Can you work these out from the drawing? Everything is in mm from the part's minimum corner. A direction names the side the tool comes from. Coordinates: 2 decimals unless noted, no trailing zeros. Loops run counter-clockwise (first coordinate to the right, second up) from the corner with the lowest first, then second, coordinate; pieces in that order, holes last.
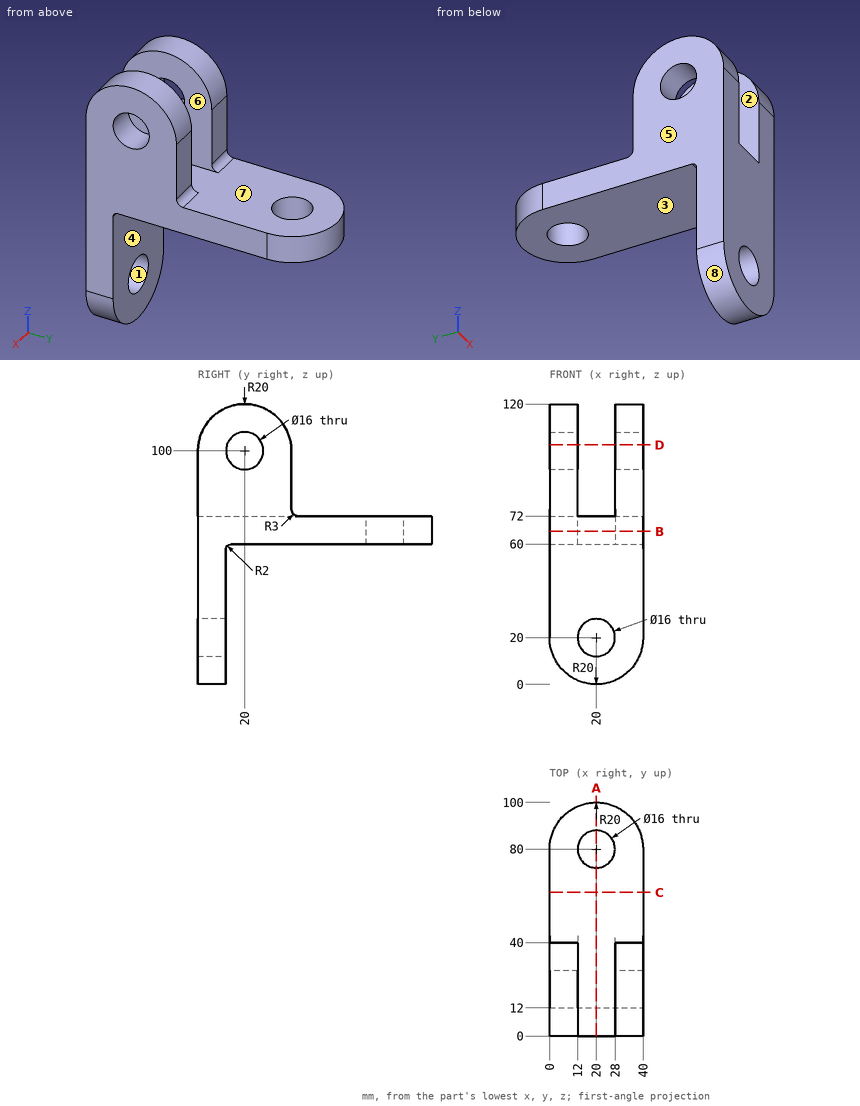
(1) Imagine slicing it at C-C, the plane y = 61.5. Write out the boundary of the cut face in (x, z).
Answers:
outline: (0, 60) - (40, 60) - (40, 72) - (0, 72) - close
(2) Imagine slicing it at D-D, the plane z = 102.5. Write out the boundary of the cut face in (x, y), and give its area (3 significant figures).
Answers:
outline: (0, 0.16) - (12, 0.16) - (12, 12.4) - (0, 12.4) - close; (0, 27.6) - (12, 27.6) - (12, 39.84) - (0, 39.84) - close; (28, 0.16) - (40, 0.16) - (40, 12.4) - (28, 12.4) - close; (28, 27.6) - (40, 27.6) - (40, 39.84) - (28, 39.84) - close
area: 588 mm2
(3) We'd pull the mould along Z, two halves only. Please class the marked faces 1, 2 and 3: +Z half, -Z half, draft (parallel to the pull), parting line (faces both ways), or undercut.
Answers:
face 1: undercut
face 2: draft
face 3: -Z half
(4) I need wall thicknesses on probe 1 along X at (y, z) = (33.5, 85.5); probe 2 along Z at (x, y) = (30.5, 66); probe 3 along Z at (x, y) = (26, 11). Which ranges of each line are inside material? Lowest first, please.
Answers:
probe 1: x = 0 to 12, 28 to 40
probe 2: z = 60 to 72
probe 3: z = 0.92 to 14.71, 25.29 to 72
(5) For pin 1 (20 mm diameter, centred on x = 10.5, y = 57.5, fed in from +Z); pin 2 (6 mm diameter, centred on x = 32, z = 84.5, fed in from +Y); pin 3 (12 mm diameter, centred on x = 24, z = 38, fed in from +Y), each with a flat end and sliding along its axis, tell me the tip position at first contact or that it passes through.
Answers:
pin 1: stops at z = 72
pin 2: stops at y = 40
pin 3: stops at y = 12
(6) Imagine slicing it at B-B, the plane z = 65.5. Write out the boundary of the cut face in (x, y).
Answers:
outline: (0, 0) - (40, 0) - (40, 80) arc R20 ccw to (0, 80) - close; hole circle Ø16 at (20, 80)
(7) Imagine slicing it at A-A, the plane x = 20. Write out the boundary of the cut face in (y, z), and give its area (3 significant figures).
Answers:
outline: (0, 0) - (12, 0) - (12, 12) - (0, 12) - close; (0, 28) - (12, 28) - (12, 58) arc R2 cw to (14, 60) - (72, 60) - (72, 72) - (0, 72) - close; (88, 60) - (100, 60) - (100, 72) - (88, 72) - close
area: 1,540 mm2
(8) Which directions (+Z, -Z, +X, -X, +Y, -Y) give clear straight access to the entire face, cutting with the end or side of a thin tool? Please do the marked faces 4, 5, 6, 7 and 8.
Answers:
face 4: -Z, +X, -X, +Y
face 5: +Z, -Z, -X, +Y, -Y
face 6: +Z, +Y, -Y
face 7: +Z, +Y
face 8: -Z, +Y, -Y
